Check sheet for the modelled part. Datum: model origin and axes. Units: mm. A direction names the side the tool comes from. Round coordinates to 2 decimals unless told otherwise and drop trailing zeros. Write each loop counter-clockwise with the first axis right and the second up, starting at its lowest first coordinate (ties: lowest second). Pieces come first, ordered by that corner, then holes. Notation, with made-up numbers: (-36, -13) -> (-16, -13) arc R20 ccw to (-16, 3) -> close; hole circle Ø1 at (-24, 79). An arc over 180 degrees is marked (long way). One line per item, written item: value.
from build123d import *
from build123d.topology import SkipClean

# Parameters (mm, degrees)
BOSS_EXTRUDE1_DEPTH    = 115.8875
SHELL1_T               = -2.54
FILLET7_R              = 1.5875
FILLET6_R              = 3.175
CUT_EXTRUDE1_DEPTH     = 1.905
FILLET8_R              = 1.5875
LPATTERN1_COUNT        = 4
LPATTERN1_PITCH        = 29.21
FILLET8_OF_LPATTERN1_R = 1.5875
LPATTERN2_COUNT        = 4
LPATTERN2_PITCH        = 29.21
FILLET8_OF_LPATTERN2_R = 1.5875
BOSS_EXTRUDE2_DEPTH    = 2.54
SKETCH5_R              = 7.385
CUT_EXTRUDE2_DEPTH     = 4.8
FILLET4_R              = 0.254
FILLET5_R              = 0.254
SKETCH6_R              = 3.2385
CUT_EXTRUDE3_DEPTH     = 278.093208583


with BuildPart() as part:
    # Sketch1 → Boss-Extrude1 (new, symmetric)
    with BuildSketch(Plane(origin=(0, 0, 0), x_dir=(0, 0, -1), z_dir=(1, 0, 0))):
        with BuildLine():
            Line((0, 0), (0, 84.901644013))
            ThreePointArc((0, 84.901644013), (1.29607654, 87.021254856), (3.773438424, 86.833524691))
            Line((3.773438424, 86.833524691), (124.268628317, 0))
            Line((124.268628317, 0), (107.976719942, 0))
            Line((107.976719942, 0), (29.650004929, 56.445280082))
            ThreePointArc((29.650004929, 56.445280082), (16.437408213, 57.446507626), (9.525, 46.141916466))
            Line((9.525, 46.141916466), (9.525, 0))
            Line((9.525, 0), (0, 0))
        make_face()
    extrude(amount=BOSS_EXTRUDE1_DEPTH, both=True)

    # Shell1
    shell1_openings = [part.faces().sort_by_distance(p)[0] for p in [
        (0, 28.222640041, -68.813362436),
        (0, 57.446507626, -16.437408213),
        (0, 23.070958233, -9.525),
    ]]
    offset(amount=SHELL1_T, openings=shell1_openings, kind=Kind.INTERSECTION)

    # Fillet7
    fillet7_edges = [part.edges().sort_by_distance(p)[0] for p in [
        (0, 84.591566193, -2.54),
    ]]
    fillet(fillet7_edges, radius=FILLET7_R)

    # Fillet6
    fillet6_edges = [part.edges().sort_by_distance(p)[0] for p in [
        (0, 2.54, -116.399469423),
    ]]
    fillet(fillet6_edges, radius=FILLET6_R)

    # Sketch3 → Cut-Extrude1 (cut, symmetric)
    with BuildSketch(Plane(origin=(0, -2.413, -15.875), x_dir=(0, 0, 1), z_dir=(-1, 0, 0))):
        with BuildLine():
            Line((-7.926699104, 71.361902399), (-8.271161087, 70.883874176))
            ThreePointArc((-8.271161087, 70.883874176), (3.476459724, 61.284711128), (15.828327064, 70.09276989))
            ThreePointArc((15.828327064, 70.09276989), (15.901291869, 70.288577921), (15.970972384, 70.485578616))
            Line((15.970972384, 70.485578616), (17.531294258, 75.017082374))
            Line((17.531294258, 75.017082374), (17.531294258, 94.003784079))
            Line((17.531294258, 94.003784079), (-8.281098949, 75.779023692))
            ThreePointArc((-8.281098949, 75.779023692), (-8.301253168, 73.554628688), (-7.926699104, 71.361902399))
        make_face()
    cut_extrude1 = extrude(amount=CUT_EXTRUDE1_DEPTH, both=True, mode=Mode.SUBTRACT)

    # Fillet8
    fillet8_edges = [part.edges().sort_by_distance(p)[0] for p in [
        (0, 72.101660209, -24.21622034),
    ]]
    fillet(fillet8_edges, radius=FILLET8_R)

    # LPattern1: Cut-Extrude1 ×4
    with Locations(*[(i * LPATTERN1_PITCH, 0, 0) for i in range(1, LPATTERN1_COUNT)]):
        add(cut_extrude1, mode=Mode.SUBTRACT)

    # Fillet8 of LPattern1
    fillet8_of_lpattern1_edges = [part.edges().sort_by_distance(p)[0] for p in [
        (29.21, 72.101660209, -24.21622034),
        (58.42, 72.101660209, -24.21622034),
        (87.63, 72.101660209, -24.21622034),
    ]]
    fillet(fillet8_of_lpattern1_edges, radius=FILLET8_OF_LPATTERN1_R)

    # LPattern2: Cut-Extrude1 ×4
    with Locations(*[(-i * LPATTERN2_PITCH, 0, 0) for i in range(1, LPATTERN2_COUNT)]):
        add(cut_extrude1, mode=Mode.SUBTRACT)

    # Fillet8 of LPattern2
    fillet8_of_lpattern2_edges = [part.edges().sort_by_distance(p)[0] for p in [
        (-29.21, 72.101660209, -24.21622034),
        (-58.42, 72.101660209, -24.21622034),
        (-87.63, 72.101660209, -24.21622034),
    ]]
    fillet(fillet8_of_lpattern2_edges, radius=FILLET8_OF_LPATTERN2_R)

    # Sketch4 → Boss-Extrude2 (add)
    with BuildSketch(Plane(origin=(115.8875, 0, 0), x_dir=(0, 0, -1), z_dir=(1, 0, 0))):
        with BuildLine():
            Line((4.7625, 80.250476708), (4.7625, 78.187860591))
            ThreePointArc((4.7625, 78.187860591), (5.681515336, 78.604108973), (6.648686934, 78.891216974))
            Line((6.648686934, 78.891216974), (4.7625, 80.250476708))
        make_face()
        with BuildLine():
            Line((30.872562622, 61.434549123), (15.608650064, 72.434318733))
            ThreePointArc((15.608650064, 72.434318733), (12.367009719, 65.545693058), (4.7625, 65.181237654))
            Line((4.7625, 65.181237654), (4.7625, 61.434549123))
            Line((4.7625, 61.434549123), (30.872562622, 61.434549123))
        make_face()
    extrude(amount=BOSS_EXTRUDE2_DEPTH)

    # Sketch5 → Cut-Extrude2 (cut)
    with SkipClean():  # the faces are left unmerged after this step: merging them gives an invalid solid
        with BuildSketch(Plane(origin=(115.8875, 0, 0), x_dir=(0, 0, -1), z_dir=(1, 0, 0))):
            with Locations(Location((8.26180921, 71.684549123, 0), (0, 0, 219.214186209))):
                Circle(SKETCH5_R)
        extrude(amount=-CUT_EXTRUDE2_DEPTH, mode=Mode.SUBTRACT)

    # Fillet4
    fillet4_edges = [part.edges().sort_by_distance(p)[0] for p in [
        (118.4275, 79.570846841, -5.705593467),
        (118.4275, 79.219168649, -4.7625),
        (118.4275, 78.604108973, -5.681515336),
    ]]
    fillet(fillet4_edges, radius=FILLET4_R)

    # Fillet5
    fillet5_edges = [part.edges().sort_by_distance(p)[0] for p in [
        (118.4275, 61.434549123, -17.817531311),
        (118.4275, 66.934433928, -23.240606343),
        (118.4275, 65.545693058, -12.367009719),
        (118.4275, 63.307893389, -4.7625),
    ]]
    fillet(fillet5_edges, radius=FILLET5_R)

    # Sketch6 → Cut-Extrude3 (cut, through all)
    with BuildSketch(Plane(origin=(-113.3475, 0, 0), x_dir=(0, 0, -1), z_dir=(1, 0, 0))):
        with Locations((8.26180921, 71.684549123)):
            Circle(SKETCH6_R)
    extrude(amount=-CUT_EXTRUDE3_DEPTH, mode=Mode.SUBTRACT)


solid = part.part
Item 1: Tool access check on faces 4 (the flat face through (-115.888, 47, -44)), 5 (the cylindrical face through (1.59, 4.79, -109.6)). Record the directions out of +Z, -Z, +X, -X, +Y, -Y that give a thin tool (end or side, any length) a straight path to the whole face; none if there is none.
Answer:
face 4: +Z, -Z, -X, +Y, -Y
face 5: none
Item 2: Sectioned sample at A-A on y = 32. Enter the section's corners in (x, z) (1 decimal).
Answer:
outline: (-115.9, -79.9) -> (115.9, -79.9) -> (115.9, -63.6) -> (113.3, -63.6) -> (113.3, -75.5) -> (-113.3, -75.5) -> (-113.3, -63.6) -> (-115.9, -63.6) -> close; (-115.9, -9.5) -> (-113.3, -9.5) -> (-113.3, -2.5) -> (113.3, -2.5) -> (113.3, -9.5) -> (115.9, -9.5) -> (115.9, 0) -> (-115.9, 0) -> close
Item 3: Depth check by flat-ended pin: P1, Ø1.5, axis at x = -53.5, y = 67.5, coming from the -Z side; P2, Ø3.5, axis at x = -37.5, z = -6, coming from the +Y side; P3, Ø14, axis at x = -41.5, y = 28.5, coming from the -Z side; P4, Ø5, axis at y = 71.68, z = -8.26, coming from the -X side. Enter the tip coordinate at first touch or a pass-through.
Answer:
P1: stops at z = -31.64
P2: stops at y = 86.49
P3: stops at z = -94.43
P4: passes through
Item 4: Sectioned sample at C-C on z = -85. Enter the section's corners in (x, y).
Answer:
outline: (-115.89, 16.56) -> (-113.35, 16.56) -> (-113.35, 25.17) -> (113.35, 25.17) -> (113.35, 16.56) -> (115.89, 16.56) -> (115.89, 28.3) -> (-115.89, 28.3) -> close
Item 5: Mould release check, pull along Y, two halves, no side actions. Record for faces 1 (the flat face through (-113.348, 49, -44)), 2 (the flat face through (1.905, 80, -10)), 3 (the flat face through (1.622, 44.025, -63.178)): pulls with the +Y half, pulls with the -Y half, needs draft (parallel to the pull), parting line crosses it, or undercut.
Answer:
face 1: undercut
face 2: needs draft
face 3: pulls with the +Y half
Item 6: Thickness scan on line 1 (X direction, y = 62, z = -17.5); line 2 (X direction, y = 32, z = -75); line 3 (Z direction, x = 91, y = 11). Record the ranges inside material, lowest first.
Answer:
line 1: x = -115.89 to -113.35, 113.35 to 118.43
line 2: x = -115.89 to -113.35, 113.35 to 115.89
line 3: z = -109 to -104.66, -2.54 to 0
